Check sheet for the modelled part. Datum: model origin and axes. Units: mm. Face numbers are marked on the shaded views. Round coordinates to 2 decimals unless told otherwise and drop trailing zeros. Order: outer loops, then holes, each group sorted by start corner. A loop starts at its lowest first (then second) coordinate and runs counter-clockwise, first axis right, second up.
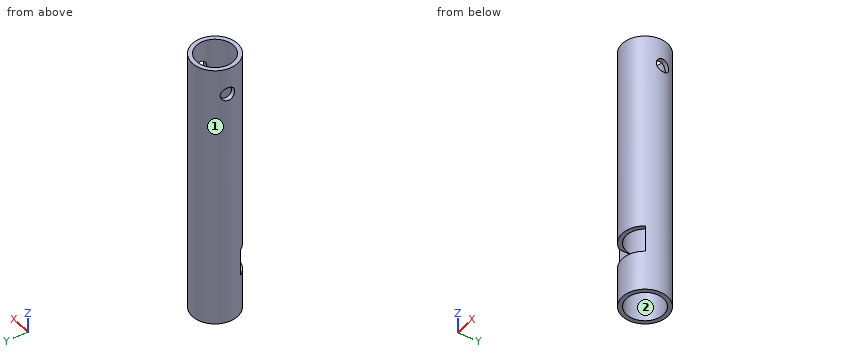
from build123d import *

# Parameters (mm, degrees)
SKETCH1_R               = 10.715625
SKETCH1_R_2             = 8.73125
BOSS_EXTRUDE1_DEPTH     = 127
SKETCH2_W               = 17.78
SKETCH2_H               = 12.7
CUT_EXTRUDE1_DEPTH      = 128.900935252
CUT_EXTRUDE2_DEPTH      = 128.900935252
CUT_EXTRUDE2_DEPTH_BACK = 128.900935252
SKETCH5_R               = 3.175


with BuildPart() as part:
    # Sketch1 → Boss-Extrude1 (new body)
    with BuildSketch(Plane.XY):
        Circle(SKETCH1_R)
        Circle(SKETCH1_R_2, mode=Mode.SUBTRACT)
    extrude(amount=BOSS_EXTRUDE1_DEPTH)

    # Sketch2 → Cut-Extrude1 (cut, through all)
    with BuildSketch(Plane(origin=(0, 0, 0), x_dir=(1, 0, 0), z_dir=(0, 1, 0))):
        with Locations((0, -25.4)):
            Rectangle(SKETCH2_W, SKETCH2_H)
    extrude(amount=-CUT_EXTRUDE1_DEPTH, mode=Mode.SUBTRACT)

    # Sketch5 → Cut-Extrude2 (cut, two sides: drawn at the far end of the back side and taken through both)
    with BuildSketch(Plane(origin=(0, 0, 0), x_dir=(0, 0, -1), z_dir=(1, 0, 0)).offset(-CUT_EXTRUDE2_DEPTH_BACK)):
        with Locations((-114.3, 1.190625)):
            Circle(SKETCH5_R)
    extrude(amount=CUT_EXTRUDE2_DEPTH + CUT_EXTRUDE2_DEPTH_BACK, mode=Mode.SUBTRACT)


solid = part.part
1) Sectioned sample at C-C on z = 16. Record the cut outline in (x, y).
2) Scan lines: line 1 (Y direction, x = 0, z = 88); line 2 (Z direction, x = 6.75, y = -6.25); line 3 (X direction, y = 3.75, z = 99). Record each from-to range of solid material in increasing order.
3) Draft check along X on the marked faces 1 and 2. Enter one of: pulls with the +X half, pulls with the -X half, needs draft (parallel to the pull), parting line crosses it, or undercut.
4) Gauge pin test, flat ends, axial feed: pin 1 (1 mm diameter, centred on y = -1, z = 33.5, fed in from -X); pin 2 (2 mm diameter, centred on x = -2, z = 40.5, fed in from -Y); pin 3 (2 mm diameter, centred on y = 2.5, z = 28, fed in from -X). Record the tip position at first contact, or that the pin passes through.
5) Sectioned sample at D-D on z = 114.3. Record the cut outline in (x, y), and give its area (3 significant figures).
6) Sectioned sample at B-B on y = 3. Record the cut outline in (x, z), and give its area (3 significant figures).
7) Sectioned sample at A-A on x = 0. Record the cut outline in (y, z), and give its area (3 significant figures).
Values found:
1. outline: circle Ø21.43 at (0, 0); hole circle Ø17.46 at (0, 0)
2. line 1: y = -10.72 to -8.73, 8.73 to 10.72
2. line 2: z = 0 to 19.05, 31.75 to 127
2. line 3: x = -10.04 to -7.88, 7.88 to 10.04
3. face 1: parting line crosses it
3. face 2: undercut
4. pin 1: stops at x = -10.7
4. pin 2: stops at y = -10.67
4. pin 3: stops at x = -10.61
5. outline: (-10.53, -1.98) arc R10.72 ccw to (10.53, -1.98) - (8.5, -1.98) arc R8.73 cw to (-8.5, -1.98) - close; (-9.79, 4.37) - (-7.56, 4.37) arc R8.73 cw to (7.56, 4.37) - (9.79, 4.37) arc R10.72 ccw to start
5. area: 95.3 mm2
6. outline: (-10.29, 0) - (-8.2, 0) - (-8.2, 111.69) - (-10.29, 111.69) - close; (-10.29, 116.91) - (-8.2, 116.91) - (-8.2, 127) - (-10.29, 127) - close; (8.2, 0) - (10.29, 0) - (10.29, 111.69) - (8.2, 111.69) - close; (8.2, 116.91) - (10.29, 116.91) - (10.29, 127) - (8.2, 127) - close
6. area: 508 mm2
7. outline: (-10.72, 0) - (-8.73, 0) - (-8.73, 19.05) - (-10.72, 19.05) - close; (-10.72, 31.75) - (-8.73, 31.75) - (-8.73, 127) - (-10.72, 127) - close; (8.73, 0) - (10.72, 0) - (10.72, 127) - (8.73, 127) - close
7. area: 479 mm2
